Read the model definition and answer for the solid it produces. Units are mm, in the model's axes. Round coordinates to 2 decimals unless told otherwise and drop trailing zeros. Order: outer loops, then holes, each group sorted by start corner. A loop starts at its lowest first (then second) coordinate and runs counter-clockwise, first axis right, second up. Notation, with made-up numbers: (-13.5, 58.25) - (-2.5, 58.25) arc R17 cw to (-2.5, 72.25) - close; hole circle Ø3 at (57, 67.5). An arc over 180 degrees is marked (long way). Answer as a JSON object with one key per item and string values. Group by question number.
Q1. Consider line 1 (Z direction, x = -1, y = 3); line 2 (X direction, y = 2.75, z = -96); line 3 (Z direction, x = -49.5, y = 4.25). Determine where each line is inside the solid, lowest interval first.
Q2. The mould has two halves that part along Z. Classify faces 1 (the flat face through (-105, 4, 1)), 2 (the flat face through (-1, 4, -105)), 3 (the cylindrical face through (-90.672, 3.944, -0.338)): pulls with the +Z half, pulls with the -Z half, needs draft (parallel to the pull), parting line crosses it, or undercut.
Q3. A cutting plane is placed at C-C on z = -29. Determine the outline of the cut face in (x, y), and give its area (3 significant figures).
Q4. A cutting plane is placed at B-B on x = 0. Determine the outline of the cut face in (y, z), and give its area (3 significant figures).
Q5. A cutting plane is placed at A-A on z = 0. Determine the outline of the cut face in (x, y), and give its area (3 significant figures).
Q6. A cutting plane is placed at D-D on y = 4.5. Count the separate pieces of the cut face and the enclosed holes in it, and give its area (3 significant figures).
```python
from build123d import *

# Parameters (mm, degrees)
SKETCH_1_W          = 210
SKETCH_1_H          = 210
SKETCH_1_R          = 85.5
SKETCH_1_R_2        = 2.6
EXTRUDE_1_DEPTH     = 8
SKETCH_2_R          = 2.6
CUT_EXTRUDE_1_DEPTH = 10
SKETCH_3_R          = 86
CUT_EXTRUDE_2_DEPTH = 10
SKETCH_4_R          = 2.65
CUT_EXTRUDE_3_DEPTH = 149.707767114


with BuildPart() as part:
    # 草图1 → 凸台-拉伸1 (new body)
    with BuildSketch(Plane(origin=(0, 0, 0), x_dir=(1, 0, 0), z_dir=(0, 1, 0))):
        Rectangle(SKETCH_1_W, SKETCH_1_H)
        with Locations(Location((0, 0, 0), (0, 0, 270))):
            Circle(SKETCH_1_R, mode=Mode.SUBTRACT)
        with Locations(Location((0, 93.25, 0), (0, 0, 270))):
            Circle(SKETCH_1_R_2, mode=Mode.SUBTRACT)
        with Locations(Location((93.25, 0, 0), (0, 0, 270))):
            Circle(SKETCH_1_R_2, mode=Mode.SUBTRACT)
        with Locations(Location((0, -93.25, 0), (0, 0, 270))):
            Circle(SKETCH_1_R_2, mode=Mode.SUBTRACT)
        with Locations(Location((-93.25, 0, 0), (0, 0, 270))):
            Circle(SKETCH_1_R_2, mode=Mode.SUBTRACT)
    extrude(amount=EXTRUDE_1_DEPTH)

    # 草图2 → 切除-拉伸1 (cut)
    with BuildSketch(Plane(origin=(0, 8, 0), x_dir=(1, 0, 0), z_dir=(0, 1, 0))):
        with Locations(Location((65.937707346, -65.937707346, 0), (0, 0, 270))):
            Circle(SKETCH_2_R)
        with Locations(Location((95, 95, 0), (0, 0, 270))):
            Circle(SKETCH_2_R)
        with Locations(Location((-65.937707346, 65.937707346, 0), (0, 0, 270))):
            Circle(SKETCH_2_R)
        with Locations(Location((65.937707346, 65.937707346, 0), (0, 0, 270))):
            Circle(SKETCH_2_R)
        with Locations(Location((-65.937707346, -65.937707346, 0), (0, 0, 270))):
            Circle(SKETCH_2_R)
        with Locations(Location((95, -95, 0), (0, 0, 270))):
            Circle(SKETCH_2_R)
        with Locations(Location((-95, -95, 0), (0, 0, 270))):
            Circle(SKETCH_2_R)
        with Locations(Location((-95, 95, 0), (0, 0, 270))):
            Circle(SKETCH_2_R)
    extrude(amount=-CUT_EXTRUDE_1_DEPTH, mode=Mode.SUBTRACT)

    # 草图3 → 切除-拉伸2 (cut)
    with BuildSketch(Plane(origin=(0, 8, 0), x_dir=(1, 0, 0), z_dir=(0, 1, 0))):
        with Locations(Location((0, 0, 0), (0, 0, 270))):
            Circle(SKETCH_3_R)
    extrude(amount=-CUT_EXTRUDE_2_DEPTH, mode=Mode.SUBTRACT)

    # 草图4 → 切除-拉伸3 (cut, through all)
    with BuildSketch(Plane(origin=(0, 8, 0), x_dir=(1, 0, 0), z_dir=(0, 1, 0))):
        with Locations(Location((85, 85, 0), (0, 0, 270))):
            Circle(SKETCH_4_R)
        with Locations(Location((-85, -85, 0), (0, 0, 270))):
            Circle(SKETCH_4_R)
        with Locations(Location((-85, 85, 0), (0, 0, 270))):
            Circle(SKETCH_4_R)
        with Locations(Location((85, -85, 0), (0, 0, 270))):
            Circle(SKETCH_4_R)
    extrude(amount=-CUT_EXTRUDE_3_DEPTH, mode=Mode.SUBTRACT)


solid = part.part
```
Result set:
{
 "1": {"line 1": "z = -105 to -95.65, -90.85 to -85.99, 85.99 to 90.85, 95.65 to 105", "line 2": "x = -105 to -97.4, -92.6 to 92.6, 97.4 to 105", "line 3": "z = -105 to -70.33, 70.33 to 105"},
 "2": {"face 1": "needs draft", "face 2": "pulls with the -Z half", "face 3": "undercut"},
 "3": {"outline": "(-105, 0) - (-80.96, 0) - (-80.96, 8) - (-105, 8) - close; (80.96, 0) - (105, 0) - (105, 8) - (80.96, 8) - close", "area": "385 mm²"},
 "4": {"outline": "(0, -105) - (8, -105) - (8, -95.85) - (0, -95.85) - close; (0, -90.65) - (8, -90.65) - (8, -86) - (0, -86) - close; (0, 86) - (8, 86) - (8, 90.65) - (0, 90.65) - close; (0, 95.85) - (8, 95.85) - (8, 105) - (0, 105) - close", "area": "221 mm²"},
 "5": {"outline": "(-105, 0) - (-95.85, 0) - (-95.85, 8) - (-105, 8) - close; (-90.65, 0) - (-86, 0) - (-86, 8) - (-90.65, 8) - close; (86, 0) - (90.65, 0) - (90.65, 8) - (86, 8) - close; (95.85, 0) - (105, 0) - (105, 8) - (95.85, 8) - close", "area": "221 mm²"},
 "6": {"separate pieces": "1", "enclosed holes": "17", "area": "20,500 mm²"}
}
